CAD build for the part. Positions are in the model's coordinates, mm. Round coordinates to 2 decimals unless told otherwise and drop trailing zeros.
```python
from build123d import *

# Parameters (mm, degrees)
SKETCH_1_R        = 7.9375
SKETCH_1_R_2      = 3.975
EXTRUDE_1_DEPTH   = 527.05
FILLET_1_R        = 2.5
MOVE_BODY_1_ANGLE = 90.5


with BuildPart() as part:
    # 스케치1 → 보스-돌출1 (new body, symmetric)
    with BuildSketch(Plane(origin=(0, 0, 0), x_dir=(1, 0, 0), z_dir=(0, 1, 0))):
        Circle(SKETCH_1_R)
        Circle(SKETCH_1_R_2, mode=Mode.SUBTRACT)
    extrude(amount=EXTRUDE_1_DEPTH, both=True)

    # 필렛1
    fillet_1_edges = [part.edges().sort_by_distance(p)[0] for p in [
        (-7.9375, -527.05, 0),
        (-7.9375, 527.05, 0),
    ]]
    fillet(fillet_1_edges, radius=FILLET_1_R)


with BuildPart() as part_1:
    # Move Body 1: moved
    add(part.part.rotate(Axis((0, 0, 0), (0, 0, 1)), MOVE_BODY_1_ANGLE))


solid = part_1.part
```
Item 1: Flat gauge pins, fed straight in: P1, Ø4, axis at y = -7, z = 4, coming from the -X side; P2, Ø2, axis at y = 2, z = -4.5, coming from the +X side; P3, Ø5, axis at x = -320.5, z = 1, coming from the +Y side. Where does each tip first touch, or does it go through?
Answers follow:
P1: stops at x = -527.03
P2: stops at x = 527.06
P3: stops at y = 5.16
Item 2: Two-plate mould, pull along Z, no slides. Class faces 1 (the cylindrical face through (-7.33, -1.78, 7.75)), 2 (the cylindrical face through (7.39, -0.8, 3.88)): released by +Z, released by -Z, zero draft, split by the parting line, or undercut.
Answers follow:
face 1: split by the parting line
face 2: undercut
Item 3: Probe line 1 (Z direction, x = 161, y = 2); line 2 (Y direction, x = 14.5, z = -5.75); line 3 (Y direction, x = 442, z = -2). List the from-to ranges inside material, lowest first.
Answers follow:
line 1: z = -7.92 to -3.93, 3.93 to 7.92
line 2: y = -5.35 to 5.6
line 3: y = -3.82 to 0.42, 7.29 to 11.54
